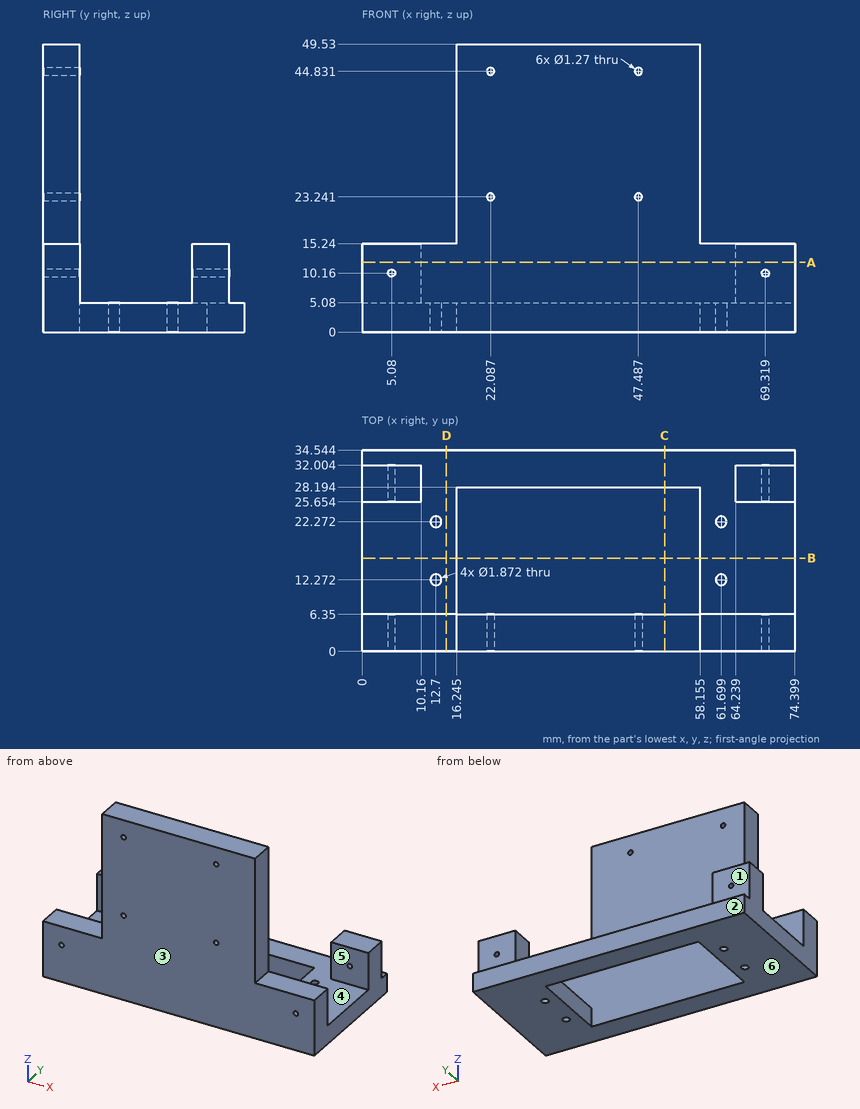
Check sheet for the drawn part. Datum: minimum x, y, z corner. Units: mm. A direction names the side the tool comes from. Round coordinates to 2 decimals unless told otherwise and drop trailing zeros. Order: outer loops, then holes, each group sorted by start corner. A loop starts at its lowest first (then second) coordinate and runs counter-clockwise, first axis right, second up.
1. Section check D-D on x = 14.5. Record the cut outline in (y, z), then the cut area to 3 significant figures.
Final values:
outline: (0, 0) - (34.54, 0) - (34.54, 5.08) - (6.35, 5.08) - (6.35, 15.24) - (0, 15.24) - close
area: 240 mm2
2. Go/stop test with flat-tipped pins: P1, Ø5, axis at x = 70, y = 28, coming from the +Z side; P2, Ø6, axis at x = 39.5, y = 10, coming from the +Z side; P3, Ø15, axis at x = 55, z = 22.5, coming from the +Y side. Record where each tip stops, or that it passes through.
Final values:
P1: stops at z = 15.24
P2: passes through
P3: stops at y = 6.35
3. Access from +Z, -Z, +X, -X, +Y, -Y to the whole of each face (thin tool, end or side, straight path). Record for the marked faces 1 and 2.
Final values:
face 1: +Z, +X, -X, +Y
face 2: +Z, -Z, +X, -X, +Y
4. Thickness scan on L1, parallel to Y at x = 12.7, z = 2.1; L2, parallel to Y at x = 64.5, z = 8.5; L3, parallel to X at y = 2, z = 10 (1 decimal). Record the ranges inside material, lowest first.
Final values:
L1: y = 0 to 11.34, 13.21 to 21.34, 23.21 to 34.54
L2: y = 0 to 6.35, 25.65 to 32
L3: x = 0 to 4.5, 5.7 to 68.7, 69.9 to 74.4
5. Release check for a two-part mould opening along Y. For the marked faces 3, 4, 5 and 6 record: +Y half, -Y half, draft (parallel to the pull), parting line (faces both ways), or undercut.
Final values:
face 3: -Y half
face 4: undercut
face 5: undercut
face 6: draft
6. Section check A-A on z = 12. Record the cut outline in (x, y).
Final values:
outline: (0, 0) - (74.4, 0) - (74.4, 6.35) - (0, 6.35) - close; (0, 25.65) - (10.16, 25.65) - (10.16, 32) - (0, 32) - close; (64.24, 25.65) - (74.4, 25.65) - (74.4, 32) - (64.24, 32) - close
7. Section check B-B on y = 16. Record the cut outline in (x, z) (1 decimal), then the cut area to 3 significant figures.
Final values:
outline: (0, 0) - (16.2, 0) - (16.2, 5.1) - (0, 5.1) - close; (58.2, 0) - (74.4, 0) - (74.4, 5.1) - (58.2, 5.1) - close
area: 165 mm2
8. Section check C-C on x = 52. Record the cut outline in (y, z), then the cut area to 3 significant figures.
Final values:
outline: (0, 0) - (6.35, 0) - (6.35, 49.53) - (0, 49.53) - close; (28.19, 0) - (34.54, 0) - (34.54, 5.08) - (28.19, 5.08) - close
area: 347 mm2
